```python
from build123d import *

# Parameters (mm, degrees)
BOSS_EXTRUDE1_DEPTH      = 1
BOSS_EXTRUDE2_DEPTH      = 3
BOSS_EXTRUDE2_DEPTH_BACK = 3
FILLET1_R                = 1


with BuildPart() as part:
    # Sketch1 → Boss-Extrude1 (new body)
    with BuildSketch(Plane(origin=(0, 0, 0), x_dir=(1, 0, 0), z_dir=(0, 1, 0))):
        with BuildLine():
            Line((-14.1, -7.5), (14.1, -7.5))
            ThreePointArc((14.1, -7.5), (15.514213562, -6.914213562), (16.1, -5.5))
            Line((16.1, -5.5), (16.1, 5.5))
            ThreePointArc((16.1, 5.5), (15.514213562, 6.914213562), (14.1, 7.5))
            Line((14.1, 7.5), (-14.1, 7.5))
            ThreePointArc((-14.1, 7.5), (-15.514213562, 6.914213562), (-16.1, 5.5))
            Line((-16.1, 5.5), (-16.1, -5.5))
            ThreePointArc((-16.1, -5.5), (-15.514213562, -6.914213562), (-14.1, -7.5))
        make_face()
        with BuildLine():
            Line((9.9, -2.5), (9.9, 2.5))
            ThreePointArc((9.9, 2.5), (11.5, 4.1), (13.1, 2.5))
            Line((13.1, 2.5), (13.1, -2.5))
            ThreePointArc((13.1, -2.5), (11.5, -4.1), (9.9, -2.5))
        make_face(mode=Mode.SUBTRACT)
        with BuildLine():
            Line((-9.9, -2.5), (-9.9, 2.5))
            ThreePointArc((-9.9, 2.5), (-11.5, 4.1), (-13.1, 2.5))
            Line((-13.1, 2.5), (-13.1, -2.5))
            ThreePointArc((-13.1, -2.5), (-11.5, -4.1), (-9.9, -2.5))
        make_face(mode=Mode.SUBTRACT)
    extrude(amount=BOSS_EXTRUDE1_DEPTH)

    # Sketch2 → Boss-Extrude2 (add, two sides: drawn at the far end of the back side and taken through both)
    with BuildSketch(Plane(origin=(0, 0, 0), x_dir=(0, 0, -1), z_dir=(1, 0, 0)).offset(-BOSS_EXTRUDE2_DEPTH_BACK)):
        with BuildLine():
            Line((6.5, 6.5), (6.5, 1))
            Line((6.5, 1), (-7.5, 1))
            Line((-7.5, 1), (0.779747183, 6.059845501))
            ThreePointArc((0.779747183, 6.059845501), (1.531550752, 6.387865691), (2.344097212, 6.5))
            Line((2.344097212, 6.5), (6.5, 6.5))
        make_face()
    extrude(amount=BOSS_EXTRUDE2_DEPTH + BOSS_EXTRUDE2_DEPTH_BACK)

    # Fillet1
    # the kernel refuses this fillet: 1 mm, written as the material it adds along each edge
    with BuildSketch(Plane(origin=(-3, 1, -6.5), x_dir=(-1, 0, 0), z_dir=(0, 0, 1))) as fillet1_piece_1_section:
        with BuildLine():
            CenterArc((FILLET1_R, -FILLET1_R), FILLET1_R, 90, 90)
            Line((0, -FILLET1_R), (0, 0))
            Line((0, 0), (FILLET1_R, 0))
        make_face()
    fillet1_piece_1 = extrude(amount=14, mode=Mode.PRIVATE)
    fillet1_piece_1 = split(fillet1_piece_1, bisect_by=Plane(origin=(-3.229666566, 4.255348718, 2.173065734), z_dir=(0, -0.8532818336519591, -0.5214500094539749)), keep=Keep.TOP, mode=Mode.PRIVATE)
    add(fillet1_piece_1)
    with BuildSketch(Plane(origin=(3, 1, -6.5), x_dir=(1, 0, 0), z_dir=(0, 0, 1))) as fillet1_piece_2_section:
        with BuildLine():
            CenterArc((FILLET1_R, FILLET1_R), FILLET1_R, 180, 90)
            Line((0, FILLET1_R), (0, 0))
            Line((0, 0), (FILLET1_R, 0))
        make_face()
    fillet1_piece_2 = extrude(amount=14, mode=Mode.PRIVATE)
    fillet1_piece_2 = split(fillet1_piece_2, bisect_by=Plane(origin=(3.229666566, 4.255348718, 2.173065734), z_dir=(0, -0.8532818336519591, -0.5214500094539749)), keep=Keep.TOP, mode=Mode.PRIVATE)
    add(fillet1_piece_2)


solid = part.part
```
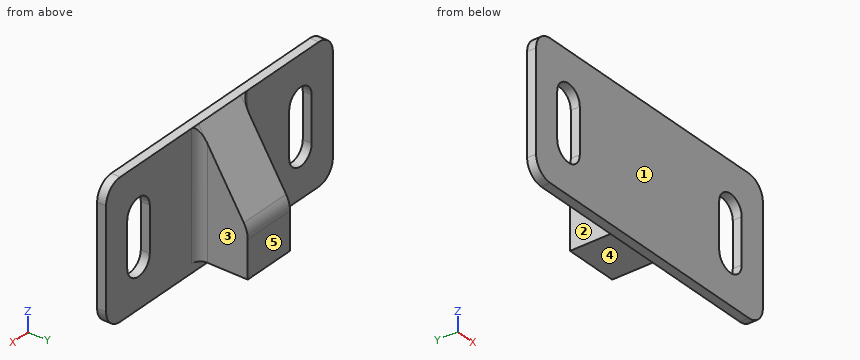
The model under review builds one solid part; all positions refer to its coordinate system, in mm. Face numbers are marked on the shaded views. A direction names the side the tool comes from. Round coordinates to 2 decimals unless told otherwise and drop trailing zeros. Write each loop counter-clockwise with the first axis right and the second up, starting at its lowest first coordinate (ties: lowest second). Pieces come first, ordered by that corner, then holes.
(1) Insertion check: pin 1 (1 mm diameter, centred on x = -5.5, z = -5, fed in from -Y); pin 2 (8 mm diameter, centred on x = 10.5, z = -4, fed in from +Y); pin 3 (4.5 mm diameter, centred on x = 0.5, z = 1, fed in from +Y). Each pin has a flat end and moves straight along its axis. Give the tip position at first contact, or say it passes through.
(2) Wall thickness on L1, parallel to Y at x = -13, z = -6.5; L2, parallel to X at y = 4, z = 0.75; L3, parallel to Z at x = 11, y = 0.75: over which ranges is each line inside the solid? List them lowest first.
(3) We need section B-B on z = 1. Give the boundary of the cut face in (x, y).
(4) Mouldability with a two-part tool opening along Z and no side actions: class the marked faces 4 and 5 as +Z half, -Z half, draft (parallel to the pull), parting line (faces both ways), or undercut.
(5) We need section D-D on y = 3.5. Give the boundary of the cut face in (x, z), and give its area (3 significant figures).
(6) We need section A-A on x = -11.5. Give the boundary of the cut face in (y, z).
(7) We need section C-C on x = 2.5. Give the boundary of the cut face in (y, z), and give its area (3 significant figures).
(8) Machinability: for the marked faces 1, 2 and 3, which of the approach directions +Z, -Z, +X, -X, +Y, -Y give a long, thin tool a straight path to every point of the face, cutting with its end or side? Answer none if there is none.
Findings below:
1. pin 1: stops at y = 0
1. pin 2: stops at y = 1
1. pin 3: stops at y = 6.29
2. L1: y = 0 to 1
2. L2: x = -3 to 3
2. L3: z = -7.5 to -4.02, 4.02 to 7.5
3. outline: (-16.1, 0) - (-13.1, 0) - (-13.1, 1) - (-16.1, 1) - close; (-9.9, 0) - (9.9, 0) - (9.9, 1) - (4, 1) arc R1 cw to (3, 2) - (3, 4.97) - (-3, 4.97) - (-3, 2) arc R1 cw to (-4, 1) - (-9.9, 1) - close; (13.1, 0) - (16.1, 0) - (16.1, 1) - (13.1, 1) - close
4. face 4: -Z half
4. face 5: draft
5. outline: (-3, -6.5) - (3, -6.5) - (3, 3.41) - (-3, 3.41) - close
5. area: 59.5 mm2
6. outline: (0, -7.5) - (1, -7.5) - (1, -4.1) - (0, -4.1) - close; (0, 4.1) - (1, 4.1) - (1, 7.5) - (0, 7.5) - close
7. outline: (0, -7.5) - (1, -7.5) - (1, -6.5) - (6.5, -6.5) - (6.5, -2.34) arc R3 ccw to (6.06, -0.78) - (1, 7.5) - (0, 7.5) - close
7. area: 67.2 mm2
8. face 1: +Z, -Z, +X, -X, -Y
8. face 2: +Z, -Z, -X, +Y
8. face 3: +Z, -Z, +X, +Y
